Can you work these out from the model? Positions are in its coordinate system, mm. A direction names the side the tool comes from. Coordinates: 2 decimals unless noted, no trailing zeros. Loops run counter-clockwise (first coordinate to the right, second up) from the corner with the lowest first, then second, coordinate; pieces in that order, holes last. Notation, with made-up numbers: M 80,-9 L 119,-9 A22 cw 119,19 Z; hole C 1.5,30 d3. An arc over 180 degrees is marked long. Answer as a JSON object with one key per item and string values. Group by question number.
Item 1: I'm going to push flat-ended pins straight in: pin 1 Ø3 at (x, z) = (61, 24.5) entering from +Y; pin 2 Ø15 at (y, z) = (37.5, 25.5) entering from +X; pin 3 Ø3 at (x, y) = (5, 69) entering from +Z; pin 4 Ø3 at (x, z) = (58.72, 12.55) entering from -Y. Where does each tip first touch, or does it pass through?
Item 2: Suppose I cut it at A-A (y = 17.5). Write out the boundary of the cut face in (x, z).
Item 3: Suppose I cut it at D-D (z = 18.5). Write out the boundary of the cut face in (x, y).
Item 4: We'd pull the mould along X, two halves only. Please class faces 4 (the flat face through (-3.282, 39, 23)), 5 (the flat face through (53.718, 42, 23)), 6 (the cylindrical face through (56.734, 2.465, 34.072)): +X half, -X half, draft (parallel to the pull), parting line (faces both ways), or undercut.
Item 5: If I drill on line 1 (Z direction, x = 6, y = 33); line 2 (X direction, y = 58, z = 38); line 3 (Y direction, x = 59, z = 39.5), over which ranges is the centre line in solid material (lowest first)?
Item 6: Which directions (+Z, -Z, +X, -X, +Y, -Y) give clear straight access to the entire face, cutting with the end or side of a thin tool? Please do faces 1 (the flat face through (25, 5, 22)), 2 (the flat face through (59, 5, 22)), 3 (the flat face through (25, 80, 44)).
Item 7: Suppose I cut it at C-C (x = 33). Write out the boundary of the cut face in (y, z), then the cut area to 4 significant figures.
Item 8: Suppose I cut it at B-B (z = 11.5). Write out the boundary of the cut face in (x, y), then the cut area to 3 significant figures.
```python
from build123d import *

# Parameters (mm, degrees)
SKETCH1_W           = 57
SKETCH1_H           = 50
BOSS_EXTRUDE1_DEPTH = 80
SKETCH2_W           = 47
SKETCH2_H           = 40
CUT_EXTRUDE1_DEPTH  = 75
SKETCH3_W           = 10
SKETCH3_H           = 50.004105979
SKETCH3_R           = 2.5
BOSS_EXTRUDE2_DEPTH = 5


with BuildPart() as part:
    # Sketch1 → Boss-Extrude1 (new body)
    with BuildSketch(Plane(origin=(0, 0, 0), x_dir=(1, 0, 0), z_dir=(0, 1, 0))):
        with Locations((25.218232044, -22.546961326)):
            Rectangle(SKETCH1_W, SKETCH1_H)
    extrude(amount=BOSS_EXTRUDE1_DEPTH)

    # Sketch2 → Cut-Extrude1 (cut)
    with BuildSketch(Plane(origin=(0, 80, 0), x_dir=(1, 0, 0), z_dir=(0, 1, 0))):
        with Locations((25.218232044, -22.546961326)):
            Rectangle(SKETCH2_W, SKETCH2_H)
    extrude(amount=-CUT_EXTRUDE1_DEPTH, mode=Mode.SUBTRACT)

    # Sketch3 → Boss-Extrude2 (add)
    with BuildSketch(Plane(origin=(0, 0, 0), x_dir=(1, 0, 0), z_dir=(0, 1, 0))):
        with Locations((58.718232044, -22.549014316)):
            Rectangle(SKETCH3_W, SKETCH3_H)
        with Locations((58.718232044, -12.551067305)):
            Circle(SKETCH3_R, mode=Mode.SUBTRACT)
        with Locations((58.718232044, -32.551067305)):
            Circle(SKETCH3_R, mode=Mode.SUBTRACT)
    extrude(amount=BOSS_EXTRUDE2_DEPTH)


solid = part.part
```
From the geometry:
{
 "1": {"pin 1": "y = 5", "pin 2": "x = 53.72", "pin 3": "z = 47.55", "pin 4": "through"},
 "2": {"outline": "M -3.28,-2.45 L 53.72,-2.45 L 53.72,47.55 L -3.28,47.55 Z; hole M 1.72,2.55 L 48.72,2.55 L 48.72,42.55 L 1.72,42.55 Z"},
 "3": {"outline": "M -3.28,0 L 63.72,0 L 63.72,5 L 53.72,5 L 53.72,80 L 48.72,80 L 48.72,5 L 1.72,5 L 1.72,80 L -3.28,80 Z"},
 "4": {"face 4": "-X half", "face 5": "+X half", "face 6": "undercut"},
 "5": {"line 1": "-2.45 to 2.55, 42.55 to 47.55", "line 2": "-3.28 to 1.72, 48.72 to 53.72", "line 3": "0 to 5"},
 "6": {"face 1": "+Y", "face 2": "+Z, -Z, +X, +Y", "face 3": "+Z, -Z, +X, -X, +Y"},
 "7": {"outline": "M 0,-2.45 L 80,-2.45 L 80,2.55 L 5,2.55 L 5,42.55 L 80,42.55 L 80,47.55 L 0,47.55 Z", "area": "1,000 mm2"},
 "8": {"outline": "M -3.28,0 L 56.45,0 L 56.45,5 L 53.72,5 L 53.72,80 L 48.72,80 L 48.72,5 L 1.72,5 L 1.72,80 L -3.28,80 Z; M 60.99,0 L 63.72,0 L 63.72,5 L 60.99,5 Z", "area": "1,060 mm2"}
}
